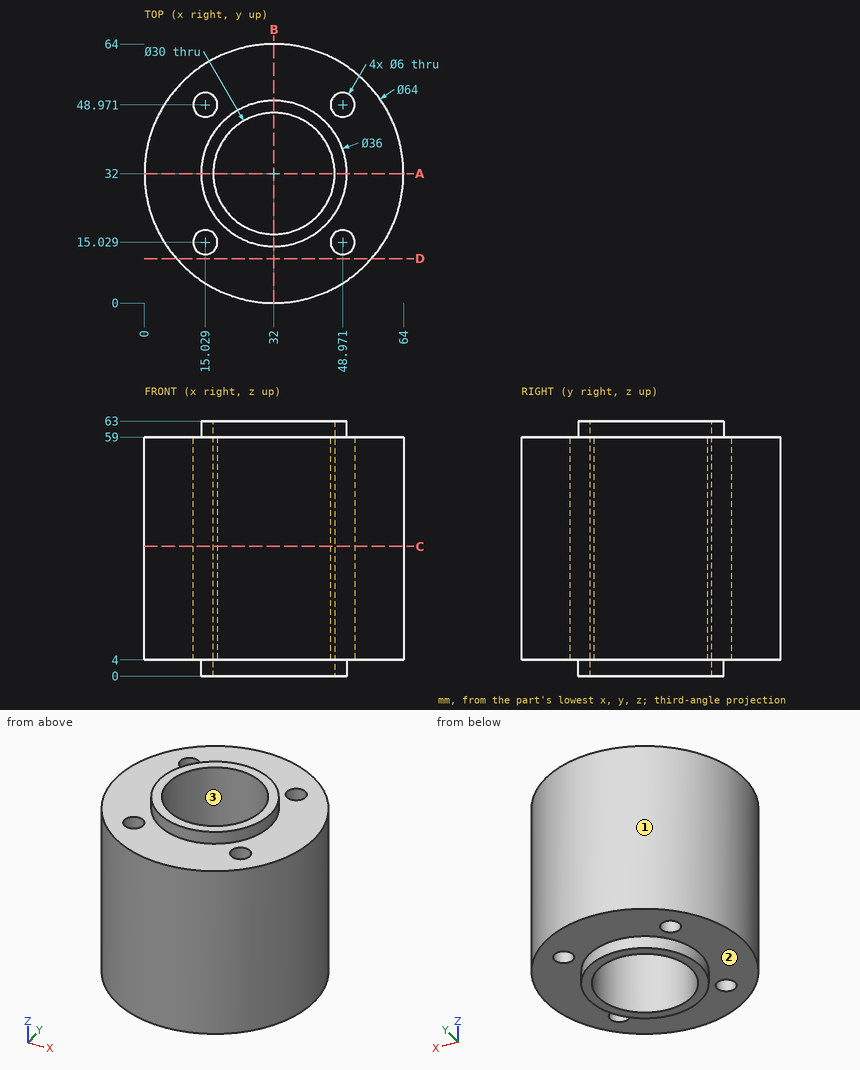
Print and shaded views of the part. All mm, measured from the part's lowest x, y and z. Give positions to 0.01 mm unless a question says otherwise; leave off trailing zeros. Order: outer loops, then holes, each group sorted by start corner. A loop starts at its lowest first (then second) coordinate and runs counter-clockwise, first axis right, second up. Notation, with made-up numbers: (-35, 59.25) - (-31, 59.25) arc R33 cw to (-31, 95.25) - close; hole circle Ø4 at (-16.5, 16). An arc over 180 degrees is marked (long way). Use a Markdown table: item, result.
1) Flat gauge pins, fed straight in: P1, Ø8, axis at x = 48.97, y = 15.03, coming from the -Z side; P2, Ø10, axis at x = 51.5, z = 22.5, coming from the +Y side; P3, Ø1, axis at y = 9.5, z = 26.5, coming from the +X side; P4, Ø5.5, axis at x = 15.03, y = 48.97, coming from the +Z side. Where does each tip first touch, or does it go through?
Checked values:
| item | result |
|---|---|
| P1 | z = 4 |
| P2 | y = 60.53 |
| P3 | x = 55.24 |
| P4 | through |
2) Saw through at A-A on y = 32. List the corners of the cut face in (x, z), plus the area to 3 significant figures.
Checked values:
| item | result |
|---|---|
| outline | (0, 4) - (14, 4) - (14, 0) - (17, 0) - (17, 63) - (14, 63) - (14, 59) - (0, 59) - close; (47, 0) - (50, 0) - (50, 4) - (64, 4) - (64, 59) - (50, 59) - (50, 63) - (47, 63) - close |
| area | 1,920 mm² |
3) Two-plate mould, pull along Y, no slides. Class the marked faces 1, 2 and 3: +Y half, -Y half, draft (parallel to the pull), parting line (faces both ways), or undercut.
Checked values:
| item | result |
|---|---|
| face 1 | parting line |
| face 2 | draft |
| face 3 | undercut |
4) Saw through at D-D on y = 11. List the corners of the cut face in (x, z) (1 decimal).
Checked values:
| item | result |
|---|---|
| outline | (7.9, 4) - (56.1, 4) - (56.1, 59) - (7.9, 59) - close |
5) Probe L1, parallel to Y at x = 13.5, z = 17.5; L2, parallel to Y at x = 32, z = 44.5. List the from-to ranges inside material, lowest first. Write a range as from..to.
Checked values:
| item | result |
|---|---|
| L1 | 5.89..12.45, 17.61..46.39, 51.55..58.11 |
| L2 | 0..17, 47..64 |
6) Saw through at C-C on z = 32. List the corners of the cut face in (x, y), plus the area to 3 significant figures.
Checked values:
| item | result |
|---|---|
| outline | circle Ø64 at (32, 32); hole circle Ø6 at (15.03, 15.03); hole circle Ø6 at (15.03, 48.97); hole circle Ø30 at (32, 32); hole circle Ø6 at (48.97, 15.03); hole circle Ø6 at (48.97, 48.97) |
| area | 2,400 mm² |
